For this review, take the finished solid that the model builds, in its own axes (mm). A direction names the side the tool comes from. Round coordinates to 2 decimals unless told otherwise and drop trailing zeros. Write each loop counter-clockwise with the first axis right and the second up, starting at its lowest first coordinate (ties: lowest second). Pieces come first, ordered by that corner, then holes.
from build123d import *

# Parameters (mm, degrees)
SKETCH1_R                    = 76.4
BOSS_EXTRUDE1_DEPTH          = 20
CUT_EXTRUDE1_REACH           = 111.881
SKETCH2_R                    = 62.5
CUT_EXTRUDE2_DEPTH           = 110.881390599
CIRPATTERN1_COUNT            = 4
R_P_TITION_CIRCULAIRE2_COUNT = 4
CUT_EXTRUDE4_START           = -20
CUT_EXTRUDE4_DEPTH           = 130.881390756
CIRPATTERN8_COUNT            = 4
CIRPATTERN8_START            = -20
CIRPATTERN8_COPY_1_DEPTH     = 130.881390756
CIRPATTERN8_COPY_2_DEPTH     = 130.881390756
CIRPATTERN8_COPY_3_DEPTH     = 130.881390756
SPLIT1_SURFACE_1_BACK        = 218.015
SPLIT1_SURFACE_1_DEPTH       = 436.03


# Read off the part's stored shape, not the designer's step: Répétition circulaire1, Répétition linéaire1
with BuildPart() as part:
    # Sketch1 → Boss-Extrude1 (new body)
    with BuildSketch(Plane.XY):
        Circle(SKETCH1_R)
    extrude(amount=BOSS_EXTRUDE1_DEPTH)

    # Sketch2 → Cut-Extrude1 (cut, up to next)
    with BuildSketch(Plane.XY.offset(20), mode=Mode.PRIVATE) as cut_extrude1_sk1:
        Circle(SKETCH2_R)
    cut_extrude1_tool1 = extrude(cut_extrude1_sk1.sketch, amount=-CUT_EXTRUDE1_REACH, mode=Mode.PRIVATE) & part.part
    add(cut_extrude1_tool1.solids().sort_by_distance((0, 0, 20))[0], mode=Mode.SUBTRACT)

    # Sketch39 → Cut-Extrude2 (cut, through all)
    with BuildSketch(Plane(origin=(0, 0, 0), x_dir=(-1, 0, 0), z_dir=(0, 0, -1))):
        with BuildLine():
            Line((-15, 70.95), (15, 70.95))
            ThreePointArc((15, 70.95), (16.95, 69), (15, 67.05))
            Line((15, 67.05), (-15, 67.05))
            ThreePointArc((-15, 67.05), (-16.95, 69), (-15, 70.95))
        make_face()
    cut_extrude2 = extrude(amount=-CUT_EXTRUDE2_DEPTH, mode=Mode.SUBTRACT)

    # CirPattern1: Cut-Extrude2 ×4 about axis
    cirpattern1_axis = Axis((0, 0, 0), (0, 0, 1))
    for i in range(1, CIRPATTERN1_COUNT):
        add(cut_extrude2.rotate(cirpattern1_axis, i * 360 / CIRPATTERN1_COUNT), mode=Mode.SUBTRACT)

    # Esquisse2 → M3 Tapped Hole1 (revolve, cut)
    with BuildSketch(Plane(origin=(49.10897338, -58.525795454, 5), x_dir=(0.766044443118979, 0.6427876096865381, 0), z_dir=(0, 0, 1))):
        Polygon((0, 0), (0, 8.751075774), (1.25, 8), (1.25, 0), align=None)
    revolve(axis=Axis((53.190674702, -63.390177668, 5), (-0.6427876096865383, 0.766044443118979, 0)), mode=Mode.SUBTRACT)

    # Esquisse2 at point 2 (carried to point 2, square into its face) → M3 Tapped Hole1 at 2 (revolve, cut)
    with BuildSketch(Plane(origin=(-54.022958083, -54.022958083, 5), x_dir=(0.707106781, -0.707106781, 0), z_dir=(0, 0, 1))):
        Polygon((0, 0), (0, 8.751075774), (1.25, 8), (1.25, 0), align=None)
    revolve(axis=Axis((-58.513086143, -58.513086143, 5), (0.707106781, 0.707106781, 0)), mode=Mode.SUBTRACT)

    # Esquisse2 at point 3 (carried to point 3, square into its face) → M3 Tapped Hole1 at 3 (revolve, cut)
    with BuildSketch(Plane(origin=(-58.525795454, 49.10897338, 5), x_dir=(-0.642788057, -0.766044068, 0), z_dir=(0, 0, 1))):
        Polygon((0, 0), (0, 8.751075774), (1.25, 8), (1.25, 0), align=None)
    revolve(axis=Axis((-63.390175285, 53.190677542, 5), (0.766044068, -0.642788057, 0)), mode=Mode.SUBTRACT)

    # Répétition circulaire1 outline → Répétition circulaire1 (revolve, cut)
    with BuildSketch(Plane(origin=(0, 0, 5), x_dir=(0.6427876096865408, 0.7660444431189769, 0), z_dir=(0, 0, -1))):
        Polygon((0, 67.648924226), (1.25, 68.4), (1.25, 76.400001412), (0, 76.400001412), align=None)
    revolve(axis=Axis((0, 0, 5), (0.7660444431189771, -0.6427876096865409, 0)), mode=Mode.SUBTRACT)

    # R_p_tition circulaire1 2 outline → R_p_tition circulaire1 2 (revolve, cut)
    with BuildSketch(Plane(origin=(0, 0, 5), x_dir=(0.707106781186546, -0.707106781186549, 0), z_dir=(0, 0, 1))):
        Polygon((0, 67.648924226), (1.25, 68.4), (1.25, 76.400001412), (0, 76.400001412), align=None)
    revolve(axis=Axis((0, 0, 5), (0.707106781186549, 0.707106781186546, 0)), mode=Mode.SUBTRACT)

    # R_p_tition circulaire1 3 outline → R_p_tition circulaire1 3 (revolve, cut)
    with BuildSketch(Plane(origin=(0, 0, 5), x_dir=(0.7660444431189789, 0.6427876096865381, 0), z_dir=(0, 0, -1))):
        Polygon((1.25, -76.400001412), (1.25, -68.4), (0, -67.648924226), (0, -76.400001412), align=None)
    revolve(axis=Axis((0, 0, 5), (0.6427876096865381, -0.7660444431189789, 0)), mode=Mode.SUBTRACT)

    # Répétition linéaire1 outline → Répétition linéaire1 (revolve, cut)
    with BuildSketch(Plane(origin=(0, 0, 15), x_dir=(0.6427876096865408, 0.7660444431189769, 0), z_dir=(0, 0, -1))):
        Polygon((1.25, -76.400001412), (1.25, -68.4), (0, -67.648924226), (0, -76.400001412), align=None)
        Polygon((0, 76.400001412), (0, 67.648924226), (1.25, 68.4), (1.25, 76.400001412), align=None)
    revolve(axis=Axis((0, 0, 15), (0.7660444431189771, -0.6427876096865409, 0)), mode=Mode.SUBTRACT)

    # R_p_tition lin_aire1 2 outline → R_p_tition lin_aire1 2 (revolve, cut)
    with BuildSketch(Plane(origin=(0, 0, 15), x_dir=(0.707106781186546, -0.707106781186549, 0), z_dir=(0, 0, 1))):
        Polygon((1.25, -76.400001412), (1.25, -68.4), (0, -67.648924226), (0, -76.400001412), align=None)
        Polygon((0, 76.400001412), (0, 67.648924226), (1.25, 68.4), (1.25, 76.400001412), align=None)
    revolve(axis=Axis((0, 0, 15), (0.707106781186549, 0.707106781186546, 0)), mode=Mode.SUBTRACT)

    # R_p_tition lin_aire1 3 outline → R_p_tition lin_aire1 3 (revolve, cut)
    with BuildSketch(Plane(origin=(0, 0, 15), x_dir=(0.7660444431189789, 0.6427876096865381, 0), z_dir=(0, 0, -1))):
        Polygon((0, 67.648924226), (1.25, 68.4), (1.25, 76.400001412), (0, 76.400001412), align=None)
        Polygon((1.25, -68.4), (0, -67.648924226), (0, -76.400001412), (1.25, -76.400001412), align=None)
    revolve(axis=Axis((0, 0, 15), (0.6427876096865381, -0.7660444431189789, 0)), mode=Mode.SUBTRACT)

    # Esquisse4 → CBORE for M6 Hex Socket Head Cap Screw1 (revolve, cut)
    with BuildSketch(Plane(origin=(0, 76.4, 10), x_dir=(0, 0, 1), z_dir=(1, 0, 0))):
        Polygon((0, 0), (0, 30.482840043), (3.3, 28.5), (3.3, 4.2), (5.5, 4.2), (5.5, 0), align=None)
    cbore_for_m6_hex_socket_head_cap_screw1 = revolve(axis=Axis((0, 82.75, 10), (0, -1, 0)), mode=Mode.SUBTRACT)

    # Répétition circulaire2: CBORE for M6 Hex Socket Head Cap Screw1 ×4 about axis
    r_p_tition_circulaire2_axis = Axis((0, 0, 0), (0, 0, 1))
    for i in range(1, R_P_TITION_CIRCULAIRE2_COUNT):
        add(cbore_for_m6_hex_socket_head_cap_screw1.rotate(r_p_tition_circulaire2_axis, i * 360 / R_P_TITION_CIRCULAIRE2_COUNT), mode=Mode.SUBTRACT)

    # Sketch47 → Cut-Extrude4 (cut)
    with BuildSketch(Plane(origin=(0, 0, 0), x_dir=(-1, 0, 0), z_dir=(0, 0, -1)).offset(CUT_EXTRUDE4_START)):
        with BuildLine():
            Line((8, 64.4), (0, 64.4))
            Line((0, 64.4), (0, 62.5))
            ThreePointArc((0, 62.5), (7.806310396, 62.010575856), (15.490361696, 60.549968576))
            ThreePointArc((15.490361696, 60.549968576), (13.852369253, 61.240856226), (12.488718209, 62.38138278))
            ThreePointArc((12.488718209, 62.38138278), (10.460864007, 63.872124664), (8, 64.4))
        make_face()
    cut_extrude4 = extrude(amount=CUT_EXTRUDE4_DEPTH, mode=Mode.SUBTRACT)

    # Mirror1: Cut-Extrude4 across plane
    add(cut_extrude4.mirror(Plane.ZY), mode=Mode.SUBTRACT)

    # CirPattern8: Cut-Extrude4 ×4 about axis
    cirpattern8_axis = Axis((0, 0, 0), (0, 0, 1))
    for i in range(1, CIRPATTERN8_COUNT):
        add(cut_extrude4.rotate(cirpattern8_axis, i * 360 / CIRPATTERN8_COUNT), mode=Mode.SUBTRACT)

    # CirPattern8 copy 1 sketch → CirPattern8 copy 1 (cut)
    with BuildSketch(Plane.YX.offset(CIRPATTERN8_START)):
        with BuildLine():
            Line((8, -64.4), (0, -64.4))
            Line((0, -64.4), (0, -62.5))
            ThreePointArc((0, -62.5), (7.806310396, -62.010575856), (15.490361696, -60.549968576))
            ThreePointArc((15.490361696, -60.549968576), (13.852369253, -61.240856226), (12.488718209, -62.38138278))
            ThreePointArc((12.488718209, -62.38138278), (10.460864007, -63.872124664), (8, -64.4))
        make_face()
    extrude(amount=CIRPATTERN8_COPY_1_DEPTH, mode=Mode.SUBTRACT)

    # CirPattern8 copy 2 sketch → CirPattern8 copy 2 (cut)
    with BuildSketch(Plane(origin=(0, 0, 0), x_dir=(-1, 0, 0), z_dir=(0, 0, -1)).offset(CIRPATTERN8_START)):
        with BuildLine():
            Line((8, -64.4), (0, -64.4))
            Line((0, -64.4), (0, -62.5))
            ThreePointArc((0, -62.5), (7.806310396, -62.010575856), (15.490361696, -60.549968576))
            ThreePointArc((15.490361696, -60.549968576), (13.852369253, -61.240856226), (12.488718209, -62.38138278))
            ThreePointArc((12.488718209, -62.38138278), (10.460864007, -63.872124664), (8, -64.4))
        make_face()
    extrude(amount=CIRPATTERN8_COPY_2_DEPTH, mode=Mode.SUBTRACT)

    # CirPattern8 copy 3 sketch → CirPattern8 copy 3 (cut)
    with BuildSketch(Plane(origin=(0, 0, 0), x_dir=(0, -1, 0), z_dir=(0, 0, -1)).offset(CIRPATTERN8_START)):
        with BuildLine():
            Line((8, -64.4), (0, -64.4))
            Line((0, -64.4), (0, -62.5))
            ThreePointArc((0, -62.5), (7.806310396, -62.010575856), (15.490361696, -60.549968576))
            ThreePointArc((15.490361696, -60.549968576), (13.852369253, -61.240856226), (12.488718209, -62.38138278))
            ThreePointArc((12.488718209, -62.38138278), (10.460864007, -63.872124664), (8, -64.4))
        make_face()
    extrude(amount=CIRPATTERN8_COPY_3_DEPTH, mode=Mode.SUBTRACT)

    # Split1: cut with a surface, the side behind it stays
    # Split1 surface: a surface, the sketch's curves swept straight by 436.03 mm
    with BuildLine(Plane(origin=(0, 0, 0), x_dir=(-1, 0, 0), z_dir=(0, 0, -1)).offset(-SPLIT1_SURFACE_1_BACK), mode=Mode.PRIVATE) as split1_surface_1_path:
        Line((73.828428705, 73.828428705), (0, 0))
        Line((0, 0), (-82.641961486, 82.641961486))
    split1_surface_1 = Shell.extrude(split1_surface_1_path.wire(), (0 * SPLIT1_SURFACE_1_DEPTH, 0 * SPLIT1_SURFACE_1_DEPTH, -1 * SPLIT1_SURFACE_1_DEPTH))
    split(bisect_by=split1_surface_1, keep=Keep.BOTTOM)


solid = part.part
(1) Mouldability with a two-part tool opening along Z and no side actions: class faces 5 (the face through (-43.7, 51.8, 5.1)), 6 (the face through (-4, 67.05, 10)), 7 (the face through (-0.8, 71.3, 0)) as pulls with the +Z half, pulls with the -Z half, needs draft (parallel to the pull), parting line crosses it, or undercut.
Geometry check:
face 5: undercut
face 6: needs draft
face 7: pulls with the -Z half
(2) We need section C-C, the plane z = 9.75. Give the boundary of the cut face in (x, y), and give its area (3 significant figures).
Geometry check:
outline: (-54.02, 54.02) - (-44.19, 44.19) arc R62.5 cw to (-15.49, 60.55) arc R6 ccw to (-12.49, 62.38) arc R6 cw to (-8, 64.4) - (-3.29, 64.4) - (-3.29, 67.05) - (-15, 67.05) arc R1.95 cw to (-15, 70.95) - (-3.29, 70.95) - (-3.29, 72.2) - (-5.49, 72.2) - (-5.49, 76.2) arc R76.4 ccw to start; (3.29, 64.4) - (8, 64.4) arc R6 cw to (12.49, 62.38) arc R6 ccw to (15.49, 60.55) arc R62.5 cw to (44.19, 44.19) - (54.02, 54.02) arc R76.4 ccw to (5.49, 76.2) - (5.49, 72.2) - (3.29, 72.2) - (3.29, 70.95) - (15, 70.95) arc R1.95 cw to (15, 67.05) - (3.29, 67.05) - close
area: 1,260 mm2
(3) For pin 1 Ø6 at (x, z) = (0.5, 6) entering from -Y; pin 2 Ø12 at (y, z) = (70.5, 16.5) entering from -X; pin 3 Ø5 at (x, z) = (25.5, 7.5) entering from +Y, all flat-tipped, find the tip position at first contact; note any pin that passes through.
Geometry check:
pin 1: stops at y = 64.4
pin 2: stops at x = -40.95
pin 3: stops at y = 72.86
(4) We need section B-B, the plane y = 69. Give the boundary of the cut face in (x, z).
Geometry check:
outline: (-32.8, 0) - (-16.95, 0) - (-16.95, 20) - (-32.8, 20) - close; (16.95, 0) - (32.8, 0) - (32.8, 20) - (16.95, 20) - close
(5) For line 1 along Z through (x, y) = (0, 71); line 2 along X through (y, z) = (53.5, 14.25); line 3 along X through (y, z) = (52.5, 5), list the stretches that pass through material, from the lowest coordinate up.
Geometry check:
line 1: z = 0 to 6.7, 13.3 to 20
line 2: x = -53.5 to -46.2, -43.59 to -32.31, 32.31 to 52.09
line 3: x = -52.5 to -45.68, -43.25 to -33.91, 33.91 to 50.73
(6) We need section A-A, the plane x = 0. Give the boundary of the cut face in (y, z).
Geometry check:
outline: (64.4, 0) - (67.05, 0) - (67.05, 6.7) - (64.4, 6.7) - close; (64.4, 13.3) - (67.05, 13.3) - (67.05, 20) - (64.4, 20) - close; (70.95, 0) - (76.4, 0) - (76.4, 4.5) - (72.2, 4.5) - (72.2, 6.7) - (70.95, 6.7) - close; (70.95, 13.3) - (72.2, 13.3) - (72.2, 15.5) - (76.4, 15.5) - (76.4, 20) - (70.95, 20) - close
(7) For faces 1 (the face through (-43.42, 52.03, 14.92)), 2 (the face through (-1.652, 74.33, 15.246)), 3 (the face through (-4, 64.4, 10)), 4 (the face through (-16.95, 69.04, 9.86)), list the 3-axis set-ups (+Z, -Z, +X, -X, +Y, -Y) from which the entire face can be reached by the end or side of a thin tool; tool diameter is ignored.
Geometry check:
face 1: none
face 2: +Y
face 3: +Z, -Z, -Y
face 4: +Z, -Z
(8) We need section D-D, the plane x = -14. Give the boundary of the cut face in (y, z), and give its area (3 significant figures).
Geometry check:
outline: (61.15, 0) - (67.05, 0) - (67.05, 20) - (61.15, 20) - close; (70.95, 0) - (75.11, 0) - (75.11, 20) - (70.95, 20) - close
area: 201 mm2
